Verification items for the finished model (mm, model axes). A direction names the side the tool comes from. Round coordinates to 2 decimals unless told otherwise and drop trailing zeros. Order: outer loops, then holes, each group sorted by start corner. A loop starts at its lowest first (then second) coordinate and runs counter-clockwise, first axis right, second up. Notation, with made-up numbers: (59.25, 24) -> (88.25, 24) arc R16 cw to (88.25, 31) -> close; hole circle Ø7 at (77.5, 68.25). An arc over 180 degrees is marked (long way). Put each result on its own line as item: value.
Autodesk Inventor part; units mm, degrees
ref_plane "РабПлоскость1" through (0, 0, 5) normal (0, 0, 1) x (1, 0, 0)
ref_plane "РабПлоскость2" through (0, 7, 0) normal (0, 1, 0) x (-1, 0, 0)
ref_plane "YZ Plane" through (0, 0, 0) normal (1, 0, 0) x (0, 1, 0)
sketch "Эскиз1" plane through (0, 0, 0) normal (0, 0, 1) x (1, 0, 0)
  circle A0 centre (0, 0) radius 7
  dimension "d0" = 14
extrude "Выдавливание1" add sketch "Эскиз1" along normal blind 5
fillet "Сопряжение1" radius 0.5 2 edges at (-7, 0, 5) (-7, 0, 0)
ref_plane "РабПлоскость1" through (0, 0, 5) normal (0, 0, 1) x (1, 0, 0)
sketch "Эскиз2" plane through (0, 0, 5) normal (0, 0, 1) x (1, 0, 0)
  circle A0 centre (0, 0) radius 3.1
  dimension "d5" = 6.2
extrude "Выдавливание2" cut sketch "Эскиз2" against normal blind 4
fillet "Сопряжение2" radius 0.5 1 edges at (-3.1, 0, 5)
ref_plane "РабПлоскость2" through (0, 7, 0) normal (0, 1, 0) x (-1, 0, 0)
sketch "Эскиз3" plane through (0, 7, 0) normal (0, 1, 0) x (-1, 0, 0)
  circle A0 centre (0, 2.7) radius 1.35
  point P0 (0, 0)
  dimension "d10" = 2.7
  dimension "d11" = 2.7
extrude "Выдавливание3" cut sketch "Эскиз3" against normal through all
thread "Резьба1"
thread "Резьба2"
properties part number "опора"
Item 1: Material ranges on L1, parallel to Z at x = 0, y = 6.05; L2, parallel to Z at x = -1.75, y = -0.5; L3, parallel to Y at x = 0.5, z = 4.35, recorded low to high. Write a range as [from, to].
Check sheet entries:
L1: z = [0, 1.35], [4.05, 5]
L2: z = [0, 1]
L3: y = [-6.98, -3.06], [3.06, 6.98]
Item 2: Section check D-D on z = 1.85. Record the boundary of the cut face in (x, y).
Check sheet entries:
outline: (-1.05, -6.92) -> (-1.05, -2.92) arc R3.1 cw to (-1.05, 2.92) -> (-1.05, 6.92) arc R7 ccw to start; (1.05, -6.92) arc R7 ccw to (1.05, 6.92) -> (1.05, 2.92) arc R3.1 cw to (1.05, -2.92) -> close
Item 3: Gauge pin test, flat ends, axial feed: pin 1 Ø1.9 at (x, y) = (-1, 1) entering from +Z; pin 2 Ø2.5 at (x, z) = (0, 2.7) entering from -Y; pin 3 Ø2 at (y, z) = (-2, 2) entering from -X; pin 4 Ø2 at (y, z) = (-4, 4) entering from +X. Record the tip position at first contact, or that the pin passes through.
Check sheet entries:
pin 1: stops at z = 1
pin 2: passes through
pin 3: stops at x = -6.93
pin 4: stops at x = 6.32
Item 4: Release check for a two-part mould opening along X. For faces 3 (the flat face through (3, -3, 5)), 4 (the cylindrical face through (1.35, -4.87, 2.76)), 5 (the cylindrical face through (3.23, 6.21, 2.47)), 6 (the flat face through (0, 0, 1)) record: +X half, -X half, draft (parallel to the pull), parting line (faces both ways), or undercut.
Check sheet entries:
face 3: draft
face 4: undercut
face 5: parting line
face 6: undercut
Item 5: Section check A-A on x = 0. Record the boundary of the cut face in (y, z), then the cut area to 3 significant figures.
Check sheet entries:
outline: (-7, 0.5) arc R0.5 ccw to (-6.5, 0) -> (6.5, 0) arc R0.5 ccw to (7, 0.5) -> (7, 1.35) -> (3.1, 1.35) -> (3.1, 1) -> (-3.1, 1) -> (-3.1, 1.35) -> (-7, 1.35) -> close; (-7, 4.05) -> (-3.1, 4.05) -> (-3.1, 4.5) arc R0.5 ccw to (-3.6, 5) -> (-6.5, 5) arc R0.5 ccw to (-7, 4.5) -> close; (3.1, 4.05) -> (7, 4.05) -> (7, 4.5) arc R0.5 ccw to (6.5, 5) -> (3.6, 5) arc R0.5 ccw to (3.1, 4.5) -> close
area: 23.8 mm^2
Item 6: Section check C-C on y = 0. Record the boundary of the cut face in (x, z), then the cut area to 3 significant figures.
Check sheet entries:
outline: (-7, 0.5) arc R0.5 ccw to (-6.5, 0) -> (6.5, 0) arc R0.5 ccw to (7, 0.5) -> (7, 4.5) arc R0.5 ccw to (6.5, 5) -> (3.6, 5) arc R0.5 ccw to (3.1, 4.5) -> (3.1, 1) -> (-3.1, 1) -> (-3.1, 4.5) arc R0.5 ccw to (-3.6, 5) -> (-6.5, 5) arc R0.5 ccw to (-7, 4.5) -> close
area: 44.9 mm^2
Item 7: Section check B-B on z = 3.45. Record the boundary of the cut face in (x, y).
Check sheet entries:
outline: (-1.12, -6.91) -> (-1.12, -2.89) arc R3.1 cw to (-1.12, 2.89) -> (-1.12, 6.91) arc R7 ccw to start; (1.12, -6.91) arc R7 ccw to (1.12, 6.91) -> (1.12, 2.89) arc R3.1 cw to (1.12, -2.89) -> close
Item 8: Tool access check on faces 1 (the flat face through (0, 0, 0)), 2 (the cylindrical face through (2.864, -1.187, 2.774)). Record the directions out of +Z, -Z, +X, -X, +Y, -Y that give a thin tool (end or side, any length) a straight path to the whole face; none if there is none.
Check sheet entries:
face 1: -Z, +X, -X, +Y, -Y
face 2: +Z
